Source: CAD feature listing. Evaluate the final solid. Frame: model axes, mm. A direction names the side the tool comes from. Give positions to 0.01 mm unless a question says otherwise; leave off trailing zeros. Write each loop counter-clockwise with the first axis right and the second up, starting at its lowest first coordinate (ties: lowest second). Pieces come first, ordered by that corner, then holes. Notation, with made-up numbers: (-22.75, 59.25) -> (24.25, 59.25) arc R15 cw to (24.25, 74.25) -> close; hole circle Ø8 at (68, -13.5). An arc over 180 degrees is marked (long way). Answer as a JSON object with one key per item and string values. Group by question number.
Item 1: Access query for faces 4 (the face through (2.285, 8.813, 4.699)), 5 (the face through (0.285, 8.806, 5.199)). Directions: +Z, -Z, +X, -X, +Y, -Y. A direction counts if a zero-diameter tool reaches every point of the face in a straight line with its end or side. Return the directions, or none.
Item 2: Section query A-A on x = 22.5. Return the cut outline in (y, z).
Item 3: Section query C-C on z = 2.7. Return the cut outline in (x, y).
Item 4: Ray query, probe 1 along X at (y, z) = (8.5, 2.7); probe 2 along Y at (x, z) = (26, 4.1); probe 3 along Z at (x, y) = (16.5, 11.75). Return the intervals inside material, ascending. Write a range as from..to.
Item 5: Pull-direction query (Y, two-part tool) for faces 1 (the face through (29.715, 8.946, 5.199)), 2 (the face through (15.17, 3.66, 4.7)), 3 (the face through (29.7, 3.16, 2.22)); classes: pulls with the +Y half, pulls with the -Y half, needs draft (parallel to the pull), parting line crosses it, or undercut.
Item 6: First-contact query: pin 1 Ø1 at (x, z) = (19, 1) entering from +Y; pin 2 Ø2.5 at (x, y) = (17, 9.5) entering from -Z; pin 3 Ø0.6 at (x, y) = (22, 14.5) entering from -Z. Flat tips, straight axial feed; report the tip coordinate or a pass-through.
Item 7: Section query B-B on y = 4.75. Return the cut outline in (x, z).
from build123d import *

# Parameters (mm, degrees)
F1_DEPTH = 5.5
F2_R     = 1
F4_DEPTH = 5
F5_W     = 12.5
F5_H     = 2.9783394848
F6_DEPTH = 3.1
F7_R     = 1


with BuildPart() as f1:
    # F0 (on Top) → F1 (new body)
    with BuildSketch(Plane.XY):
        with BuildLine():
            ThreePointArc((0, 3.8761399509), (0.2928932188, 3.1690331698), (1, 2.8761399509))
            Line((1, 2.8761399509), (29, 2.8761399509))
            ThreePointArc((29, 2.8761399509), (29.7071067812, 3.1690331698), (30, 3.8761399509))
            Line((30, 3.8761399509), (30, 13.8761399509))
            ThreePointArc((30, 13.8761399509), (29.7071067812, 14.5832467321), (29, 14.8761399509))
            Line((29, 14.8761399509), (1, 14.8761399509))
            ThreePointArc((1, 14.8761399509), (0.2928932188, 14.5832467321), (0, 13.8761399509))
            Line((0, 13.8761399509), (0, 3.8761399509))
        make_face()
    extrude(amount=F1_DEPTH)

    # F2
    f2_edges = [f1.edges().sort_by_distance(p)[0] for p in [
        (0.292893, 3.169033, 5.5),
        (15, 2.87614, 5.5),
        (29.707107, 3.169033, 5.5),
        (30, 8.87614, 5.5),
        (29.707107, 14.583247, 5.5),
        (15, 14.87614, 5.5),
        (0.292893, 14.583247, 5.5),
        (0, 8.87614, 5.5),
    ]]
    fillet(f2_edges, radius=F2_R)

    # F3 (on Top) → F4 (cut)
    with BuildSketch(Plane.XY):
        with BuildLine():
            ThreePointArc((28, 13.3761399509), (27.7071067812, 14.0832467321), (27, 14.3761399509))
            Line((27, 14.3761399509), (3, 14.3761399509))
            ThreePointArc((3, 14.3761399509), (2.2928932188, 14.0832467321), (2, 13.3761399509))
            Line((2, 13.3761399509), (2, 4.3761399509))
            ThreePointArc((2, 4.3761399509), (2.2928932188, 3.6690331698), (3, 3.3761399509))
            Line((3, 3.3761399509), (14.5, 3.3761399509))
            Line((14.5, 3.3761399509), (27, 3.3761399509))
            ThreePointArc((27, 3.3761399509), (27.7071067812, 3.6690331698), (28, 4.3761399509))
            Line((28, 4.3761399509), (28, 13.3761399509))
        make_face()
    extrude(amount=F4_DEPTH, mode=Mode.SUBTRACT)

    # F5 (on Top) → F6 (cut)
    with BuildSketch(Plane.XY):
        with Locations((20.75, 14.7778680548)):
            Rectangle(F5_W, F5_H)
    extrude(amount=F6_DEPTH, mode=Mode.SUBTRACT)

    # F7
    f7_edges = [f1.edges().sort_by_distance(p)[0] for p in [
        (15, 3.37614, 5),
        (28, 8.87614, 5),
        (2.292893, 3.669033, 5),
        (2, 8.87614, 5),
        (15, 14.37614, 5),
        (2.292893, 14.083247, 5),
        (27.707107, 14.083247, 5),
        (27.707107, 3.669033, 5),
    ]]
    fillet(f7_edges, radius=F7_R)


solid = f1.part
Worked answers:
{
 "1": {"face 4": "-Z", "face 5": "+Z, -X, +Y, -Y"},
 "2": {"outline": "(2.88, 0) -> (3.38, 0) -> (3.38, 4) arc R1 cw to (4.38, 5) -> (13.38, 5) arc R1 cw to (14.38, 4) -> (14.38, 3.1) -> (14.88, 3.1) -> (14.88, 4.5) arc R1 ccw to (13.88, 5.5) -> (3.88, 5.5) arc R1 ccw to (2.88, 4.5) -> close"},
 "3": {"outline": "(0, 3.88) arc R1 ccw to (1, 2.88) -> (29, 2.88) arc R1 ccw to (30, 3.88) -> (30, 13.88) arc R1 ccw to (29, 14.88) -> (27, 14.88) -> (27, 14.38) arc R1 cw to (28, 13.38) -> (28, 4.38) arc R1 cw to (27, 3.38) -> (3, 3.38) arc R1 cw to (2, 4.38) -> (2, 13.38) arc R1 cw to (3, 14.38) -> (14.5, 14.38) -> (14.5, 14.88) -> (1, 14.88) arc R1 ccw to (0, 13.88) -> close"},
 "4": {"probe 1": "0..2, 28..30", "probe 2": "2.88..3.38, 14.37..14.88", "probe 3": "5..5.5"},
 "5": {"face 1": "needs draft", "face 2": "undercut", "face 3": "pulls with the -Y half"},
 "6": {"pin 1": "y = 3.38", "pin 2": "z = 5", "pin 3": "z = 3.1"},
 "7": {"outline": "(0, 0) -> (2, 0) -> (2, 4) arc R1 cw to (3, 5) -> (27, 5) arc R1 cw to (28, 4) -> (28, 0) -> (30, 0) -> (30, 4.5) arc R1 ccw to (29, 5.5) -> (1, 5.5) arc R1 ccw to (0, 4.5) -> close"}
}
